Design review of the part built by this model. Coordinates are the model's own, in mm. Round coordinates to 2 decimals unless told otherwise and drop trailing zeros. Loops run counter-clockwise (first coordinate to the right, second up) from the corner with the lowest first, then second, coordinate; pieces in that order, holes last. Notation, with made-up numbers: (48.5, 34.5) - (81.5, 34.5) arc R23 cw to (81.5, 68.5) - close; hole circle Ø2 at (15, 45). An arc over 180 degrees is marked (long way). Return JSON: item names as keys, results as strings. Group by question number.
(1) We need section B-B, the plane z = 10.5. Write out the cut boundary in (x, y), and give its area (3 significant figures).
(2) We need section A-A, the plane x = 0. Write out the cut boundary in (y, z).
(3) We need section C-C, the plane y = -3.25. Write out the cut boundary in (x, z), and give its area (3 significant figures).
(4) Clearance check with flat-ended pins moving along their axes: pin 1 (1 mm diameter, centred on y = -3, z = 14, fed in from +X); pin 2 (1 mm diameter, centred on y = -4, z = -2.5, fed in from -X); pin 3 (6 mm diameter, centred on x = 0, z = 10, fed in from +Y). State where each tip first meets the part, or that it passes through.
(5) We need section D-D, the plane z = 1.5. Write out the cut boundary in (x, y), and give its area (3 significant figures).
(6) Wall thickness on L1, parallel to Z at x = 0, y = -3.5; L2, parallel to X at y = -5, z = 10; L3, parallel to Z at x = 2.5, y = -1.5: over which ranges is each line inside the solid? List them lowest first. Write a range as [from, to].
from build123d import *

# Parameters (mm, degrees)
F1_DEPTH = 7.62


with BuildPart() as f1:
    # F0 (on Front) → F1 (new body)
    with BuildSketch(Plane.XZ):
        with BuildLine():
            ThreePointArc((2.388888, 7.109375), (4.126586, 6.26269), (5.59017, 5))
            ThreePointArc((5.59017, 5), (7.006293, 7.323834), (7.5, 10))
            ThreePointArc((7.5, 10), (0, 17.5), (-7.5, 10))
            ThreePointArc((-7.5, 10), (-7.006293, 7.323834), (-5.59017, 5))
            ThreePointArc((-5.59017, 5), (-4.126586, 6.26269), (-2.388888, 7.109375))
            ThreePointArc((-2.388888, 7.109375), (-1.597524, 13.3927), (3.75, 10))
            ThreePointArc((3.75, 10), (3.3927, 8.402476), (2.388888, 7.109375))
        make_face()
        with BuildLine():
            ThreePointArc((-2.388888, 2.890625), (0, 3.75), (2.388888, 2.890625))
            ThreePointArc((2.388888, 2.890625), (4.126586, 3.73731), (5.59017, 5))
            ThreePointArc((5.59017, 5), (4.126586, 6.26269), (2.388888, 7.109375))
            ThreePointArc((2.388888, 7.109375), (0, 6.25), (-2.388888, 7.109375))
            ThreePointArc((-2.388888, 7.109375), (-4.126586, 6.26269), (-5.59017, 5))
            ThreePointArc((-5.59017, 5), (-4.126586, 3.73731), (-2.388888, 2.890625))
        make_face()
        with BuildLine():
            ThreePointArc((2.388888, 2.890625), (3.3927, 1.597524), (3.75, 0))
            ThreePointArc((3.75, 0), (-1.597524, -3.3927), (-2.388888, 2.890625))
            ThreePointArc((-2.388888, 2.890625), (-4.126586, 3.73731), (-5.59017, 5))
            ThreePointArc((-5.59017, 5), (-7.006293, 2.676166), (-7.5, 0))
            ThreePointArc((-7.5, 0), (0, -7.5), (7.5, 0))
            ThreePointArc((7.5, 0), (7.006293, 2.676166), (5.59017, 5))
            ThreePointArc((5.59017, 5), (4.126586, 3.73731), (2.388888, 2.890625))
        make_face()
        with BuildLine():
            ThreePointArc((7.5, 10), (7.006293, 7.323834), (5.59017, 5))
            ThreePointArc((5.59017, 5), (7.006293, 2.676166), (7.5, 0))
            Line((7.5, 0), (7.5, 10))
        make_face()
        with BuildLine():
            ThreePointArc((-7.5, 0), (-7.006293, 2.676166), (-5.59017, 5))
            ThreePointArc((-5.59017, 5), (-7.006293, 7.323834), (-7.5, 10))
            Line((-7.5, 10), (-7.5, 0))
        make_face()
    extrude(amount=F1_DEPTH)


solid = f1.part
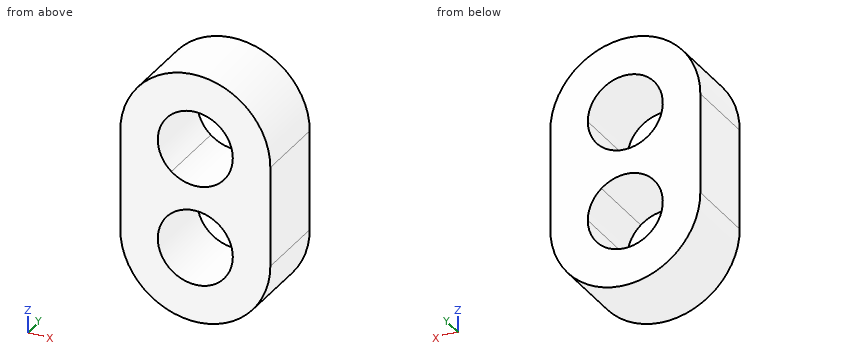
Solutions:
{
 "1": {"outline": "(-7.48, -7.62) - (-3.72, -7.62) - (-3.72, 0) - (-7.48, 0) - close; (3.72, -7.62) - (7.48, -7.62) - (7.48, 0) - (3.72, 0) - close", "area": "57.4 mm^2"},
 "2": {"outline": "(-7.62, -7.5) - (0, -7.5) - (0, -3.75) - (-7.62, -3.75) - close; (-7.62, 3.75) - (0, 3.75) - (0, 6.25) - (-7.62, 6.25) - close; (-7.62, 13.75) - (0, 13.75) - (0, 17.5) - (-7.62, 17.5) - close"},
 "3": {"outline": "(-7.5, 0) arc R7.5 ccw to (7.5, 0) - (7.5, 10) arc R7.5 ccw to (-7.5, 10) - close; hole (2.39, 2.89) arc R3.75 ccw (long way) to (3.75, 0) arc R3.75 ccw to start; hole (2.39, 7.11) arc R3.75 ccw to (3.75, 10) arc R3.75 ccw (long way) to start", "area": "238 mm^2"},
 "4": {"pin 1": "x = 6.63", "pin 2": "x = -7.23", "pin 3": "through"},
 "5": {"outline": "(-7.5, -7.62) - (-3.44, -7.62) - (-3.44, 0) - (-7.5, 0) - close; (3.44, -7.62) - (7.5, -7.62) - (7.5, 0) - (3.44, 0) - close", "area": "61.9 mm^2"},
 "6": {"L1": "[-7.5, -3.75], [3.75, 6.25], [13.75, 17.5]", "L2": "[-7.5, -3.75], [3.75, 7.5]", "L3": "[-7.07, -2.8], [2.8, 7.2], [12.8, 17.07]"}
}
